Work out the finished part from the listing and answer in its coordinate system (mm). A direction names the side the tool comes from. Coordinates: 2 decimals unless noted, no trailing zeros. Write each loop counter-clockwise with the first axis right and the second up, starting at its lowest first coordinate (ties: lowest second). Pieces come first, ordered by that corner, then holes. Notation, with made-up numbers: M 83,48 L 116,48 A20 cw 116,82 Z; hole C 57.25,69 d1. An arc over 180 degrees is marked long. Use CSV: the item, a comma, the result in double quotes.
from build123d import *

# Parameters (mm, degrees)
F0_R        = 1.5
F1_DEPTH    = 10
F2_R        = 10
F0_W        = 21.5
F0_H        = 31.25
F3_DEPTH    = 5
F4_T        = 2.5
F4_T3_DEPTH = 26.5
F4_T5_DEPTH = 10
F4_T7_DEPTH = 36.25
F5_R        = 1.5


# Not quite as in the source:
# - a shell that OpenCascade refuses in one call is made with other operations: the cavity is built on its own and cut out


with BuildPart() as f1:
    # F0 (on Front) → F1 (new body)
    with BuildSketch(Plane.XZ):
        Polygon((25.1467653117, 20.7663856067), (1.6467653117, 20.7663856067), (1.6467653117, -10.4836143933), (-19.8532346883, -10.4836143933), (-19.8532346883, -14.2336143933), (25.1467653117, -14.2336143933), align=None)
        with Locations((19.1467653117, 8.7663856067)):
            Circle(F0_R, mode=Mode.SUBTRACT)
    extrude(amount=-F1_DEPTH)

    # F2
    f2_edges = [f1.edges().sort_by_distance(p)[0] for p in [
        (25.146765, 5, 20.766386),
    ]]
    fillet(f2_edges, radius=F2_R)

    # F0 (on Front) → F3 (join)
    with BuildSketch(Plane.XZ):
        with Locations((-9.1032346883, 5.1413856067)):
            Rectangle(F0_W, F0_H)
        with BuildLine():
            ThreePointArc((-16.8532346883, 15.7663856067), (-15.6032346883, 17.0163856067), (-14.3532346883, 15.7663856067))
            Line((-14.3532346883, 15.7663856067), (-14.3532346883, 5.7663856067))
            ThreePointArc((-14.3532346883, 5.7663856067), (-15.6032346883, 4.5163856067), (-16.8532346883, 5.7663856067))
            Line((-16.8532346883, 5.7663856067), (-16.8532346883, 15.7663856067))
        make_face(mode=Mode.SUBTRACT)
        with BuildLine():
            ThreePointArc((-6.8532346883, 15.7663856067), (-5.6032346883, 17.0163856067), (-4.3532346883, 15.7663856067))
            Line((-4.3532346883, 15.7663856067), (-4.3532346883, 5.7663856067))
            ThreePointArc((-4.3532346883, 5.7663856067), (-5.6032346883, 4.5163856067), (-6.8532346883, 5.7663856067))
            Line((-6.8532346883, 5.7663856067), (-6.8532346883, 15.7663856067))
        make_face(mode=Mode.SUBTRACT)
    extrude(amount=-F3_DEPTH)

    # F4: shell of thickness 2.5, made by hand


with BuildPart() as f4_core1:
    # F4_t2: copy of F1
    add(f1.part)

    # the walls: a layer under each face that stays
    f4_faces = [f4_core1.faces().sort_by_distance(p)[0] for p in [
        (25.1467653117, 5, -1.7336143933),
        (2.6467653117, 10, 3.2663856067),
        (17.6467653117, 5, 8.7663856067),
        (-9.1032346883, 7.5, -10.4836143933),
        (-9.1032346883, 5, 5.1413856067),
        (-5.6032346883, 2.5, 4.5163856067),
        (-4.3532346883, 2.5, 10.7663856067),
        (-5.6032346883, 2.5, 17.0163856067),
        (-6.8532346883, 2.5, 10.7663856067),
        (-15.6032346883, 2.5, 4.5163856067),
        (-14.3532346883, 2.5, 10.7663856067),
        (-15.6032346883, 2.5, 17.0163856067),
        (-16.8532346883, 2.5, 10.7663856067),
        (1.6467653117, 7.5, 5.1413856067),
        (-19.8532346883, 1.6666666667, 14.9330522734),
        (9.3134319783, 8.3333333333, 20.7663856067),
        (2.6467653117, 5, -14.2336143933),
        (22.2178331235, 5, 17.8374534186),
    ]]
    thicken(f4_faces, amount=-F4_T, mode=Mode.SUBTRACT)

    # F4_s4 → F4_t3 (cut)
    with BuildSketch(Plane.YZ.offset(-22.3532346883)):
        Polygon((5.025, -10.4586143933), (5, -12.9836143933), (2.5, -12.9836143933), (2.5, -10.4836143933), align=None)
    extrude(amount=F4_T3_DEPTH, mode=Mode.SUBTRACT)

    # F4_s6 → F4_t5 (cut)
    with BuildSketch(Plane.XZ.offset(-12.5)):
        Polygon((1.6217653117, -10.4586143933), (1.6467653117, -12.9836143933), (4.1467653117, -12.9836143933), (4.1467653117, -10.4836143933), align=None)
    extrude(amount=F4_T5_DEPTH, mode=Mode.SUBTRACT)

    # F4_s8 → F4_t7 (cut)
    with BuildSketch(Plane.XY.offset(-12.9836143933)):
        Polygon((1.6217653117, 5.025), (1.6467653117, 2.5), (4.1467653117, 2.5), (4.1467653117, 5), align=None)
    extrude(amount=F4_T7_DEPTH, mode=Mode.SUBTRACT)


with BuildPart() as f1_1:
    add(f1.part)

    # what is left inside the walls is the cavity
    f4_cavity = [f4_core1.part.solids().sort_by_distance(p)[0] for p in [
        (2.646765, 0.025, -1.733614),
    ]]
    add(f4_cavity, mode=Mode.SUBTRACT)

    # F5
    f5_edges = [f1_1.edges().sort_by_distance(p)[0] for p in [
        (-19.853235, 2.5, 20.766386),
    ]]
    fillet(f5_edges, radius=F5_R)


solid = f1_1.part
Item 1: The part is cut by section D-D (z = 0.5). Write down the section's boundary in (x, y), then the cut area to 3 significant figures.
Answer:
outline,"M -19.85,0 L -17.35,0 L -17.35,2.5 L 4.15,2.5 L 4.15,7.5 L 22.65,7.5 L 22.65,0 L 25.15,0 L 25.15,10 L 1.65,10 L 1.65,5 L -19.85,5 Z"
area,"150 mm2"
Item 2: Consider probe 1 along X at (y, z) = (2.25, -1); probe 2 along Z at (x, y) = (1, 1.75); probe 3 along X at (y, z) = (2.75, 0.5). Determine where each line is inside the solid, lowest interval first.
Answer:
probe 1,"x = -19.85 to -17.35, 22.65 to 25.15"
probe 2,"z = -14.23 to -11.73, 18.27 to 20.77"
probe 3,"x = -19.85 to 4.15, 22.65 to 25.15"
Item 3: The part is cut by section B-B (x = 14.5). Write down the section's boundary in (y, z), then the cut area to 3 significant figures.
Answer:
outline,"M 0,-14.23 L 10,-14.23 L 10,20.77 L 0,20.77 L 0,18.27 L 7.5,18.27 L 7.5,-11.73 L 0,-11.73 Z"
area,"125 mm2"
Item 4: The part is cut by section A-A (z = 16.5). Write down the section's boundary in (x, y), then the cut area to 3 significant figures.
Answer:
outline,"M -19.85,0 L -16.62,0 L -16.62,5 L -19.85,5 Z; M -14.59,0 L -11.93,0 L -11.93,2.5 L -9.28,2.5 L -9.28,0 L -6.62,0 L -6.62,5 L -14.59,5 Z; M -4.59,0 L -1.93,0 L -1.93,2.5 L 4.15,2.5 L 4.15,7.5 L 19.98,7.5 L 19.98,0 L 23.34,0 L 23.34,10 L 1.65,10 L 1.65,5 L -4.59,5 Z"
area,"164 mm2"
Item 5: For a pull along X with two mould halves and no side action, classify faces 6 (the face through (-9, 5, 5)), 7 (the face through (-19.425, 2.535, 20.315)), 8 (the face through (-15.576, 2.465, 4.517)), 9 (the face through (-2.1, 1.2, 17.1)) as released by +X, released by -X, zero draft, split by the parting line, or undercut.
Answer:
face 6,"zero draft"
face 7,"released by -X"
face 8,"undercut"
face 9,"undercut"
Item 6: A tool of negligible diameter and unlimited length cuts with its end or side. For faces 1 (the face through (22.14, 5.07, 17.915)), 2 (the face through (1.647, 7, 5)), 3 (the face through (-6.853, 2, 11)), 4 (the face through (4.147, 5, 3)), 5 (the face through (2, 5, -14.234)), from which of +Z, -Z, +X, -X, +Y, -Y can it reach the whole face along a straight path? Write none if from no direction.
Answer:
face 1,"+Z, +X, +Y, -Y"
face 2,"+Z, -X, +Y"
face 3,"+Y, -Y"
face 4,"-Y"
face 5,"-Z, +X, -X, +Y, -Y"
Item 7: Given pin 1 (11 mm diameter, centred on x = -11.5, z = 0, fed in from -Y); pin 2 (4 mm diameter, centred on x = -12, y = 8, fed in from +Z); pin 3 (2 mm diameter, centred on x = -10.5, z = 2.5, fed in from +Y); pin 4 (5.5 mm diameter, centred on x = 14, z = -1, fed in from -Y), each flat-ended and moving along its own axis, determine where each tip first touches the part or whether it passes through.
Answer:
pin 1,"stops at y = 0"
pin 2,"stops at z = -10.48"
pin 3,"stops at y = 5"
pin 4,"stops at y = 7.5"
Item 8: The part is cut by section C-C (y = 1.75). Count the separate pieces of the cut face and the enclosed holes in it, then the cut area to 3 significant figures.
Answer:
separate pieces,"1"
enclosed holes,"4"
area,"547 mm2"
